For this review, use the dimensioned drawing (mm, ordinates from the lowest corner) and the shaded views. A direction names the side the tool comes from. Round coordinates to 2 decimals unless told otherwise and drop trailing zeros. Write each loop counter-clockwise with the first axis right and the second up, starting at its lowest first coordinate (ties: lowest second). Pieces come first, ordered by that corner, then holes.
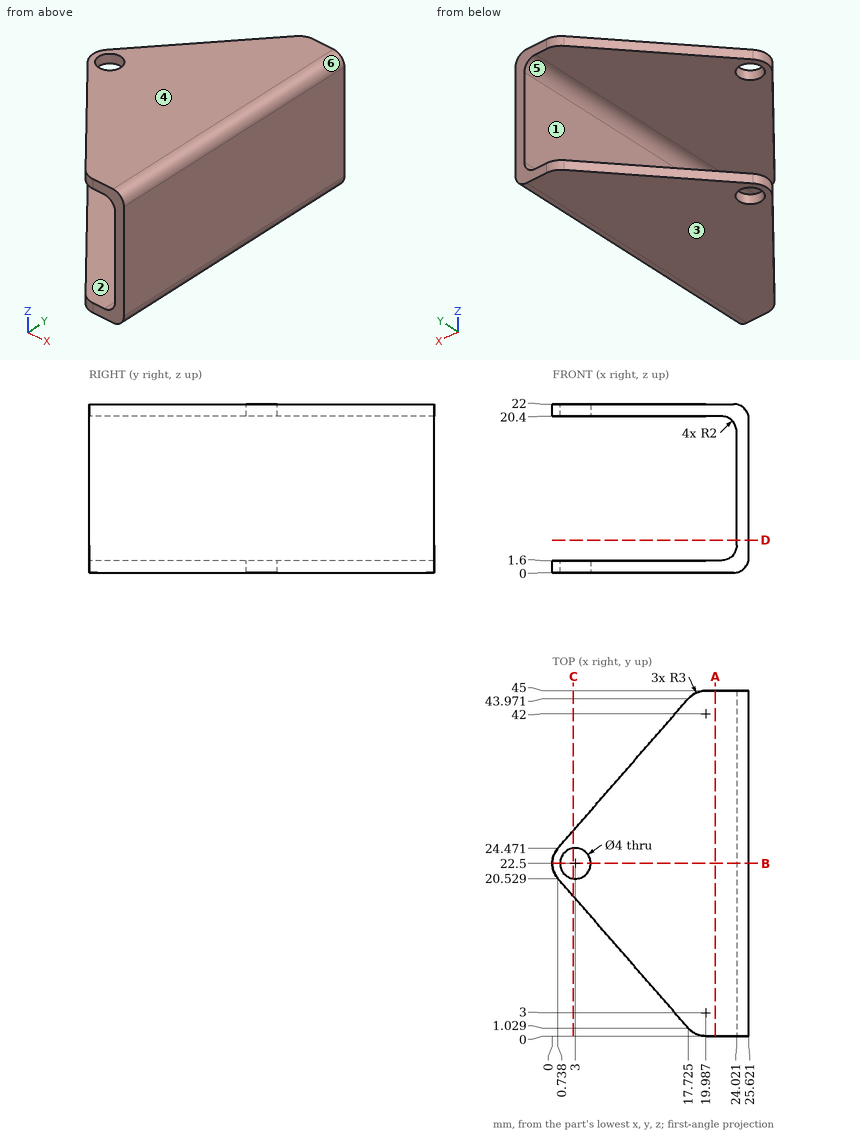
(1) We need section D-D, the plane z = 4.25. Give the boundary of the cut face in (x, y).
Geometry check:
outline: (24.02, 0) - (25.62, 0) - (25.62, 45) - (24.02, 45) - close
(2) For the marked faces 5 and 6, list the 3-axis set-ups (+Z, -Z, +X, -X, +Y, -Y) from which the entire face can be reached by the end or side of a thin tool; tool diameter is ignored.
Geometry check:
face 5: -X, +Y, -Y
face 6: +Z, +X, +Y, -Y
(3) For line 1 along Z through (x, y) = (5, 18); line 2 along X through (y, z) = (40.5, 8.25); line 3 along Z through (x, y) = (23.5, 9.5) (1 decimal), list the stretches that pass through material, from the lowest coordinate up.
Geometry check:
line 1: z = 0 to 1.6, 20.4 to 22
line 2: x = 24.02 to 25.62
line 3: z = 0 to 2.3, 19.7 to 22
(4) We need section A-A, the plane x = 21.25. Give the boundary of the cut face in (y, z), and give its area (3 significant figures).
Geometry check:
outline: (0, 0) - (45, 0) - (45, 1.6) - (0, 1.6) - close; (0, 20.4) - (45, 20.4) - (45, 22) - (0, 22) - close
area: 144 mm2
(5) For pin 1 Ø3 at (y, z) = (8, 12.5) entering from -X, flat-tipped, find the tip position at first contact; note if it passes through.
Geometry check:
pin 1: stops at x = 24.02
(6) Mouldability with a two-part tool opening along Z and no side actions: class the marked faces 1, 2, 3 and 4 as pulls with the +Z half, pulls with the -Z half, needs draft (parallel to the pull), parting line crosses it, or undercut.
Geometry check:
face 1: undercut
face 2: undercut
face 3: pulls with the -Z half
face 4: pulls with the +Z half
(7) We need section B-B, the plane y = 22.5. Give the boundary of the cut face in (x, z).
Geometry check:
outline: (0, 0) - (1, 0) - (1, 1.6) - (0, 1.6) - close; (0, 20.4) - (1, 20.4) - (1, 22) - (0, 22) - close; (5, 0) - (23.62, 0) arc R2 ccw to (25.62, 2) - (25.62, 20) arc R2 ccw to (23.62, 22) - (5, 22) - (5, 20.4) - (22.02, 20.4) arc R2 cw to (24.02, 18.4) - (24.02, 3.6) arc R2 cw to (22.02, 1.6) - (5, 1.6) - close
(8) We need section C-C, the plane x = 2.75. Give the boundary of the cut face in (y, z) (1 decimal).
Geometry check:
outline: (18.2, 0) - (20.5, 0) - (20.5, 1.6) - (18.2, 1.6) - close; (18.2, 20.4) - (20.5, 20.4) - (20.5, 22) - (18.2, 22) - close; (24.5, 0) - (26.8, 0) - (26.8, 1.6) - (24.5, 1.6) - close; (24.5, 20.4) - (26.8, 20.4) - (26.8, 22) - (24.5, 22) - close
